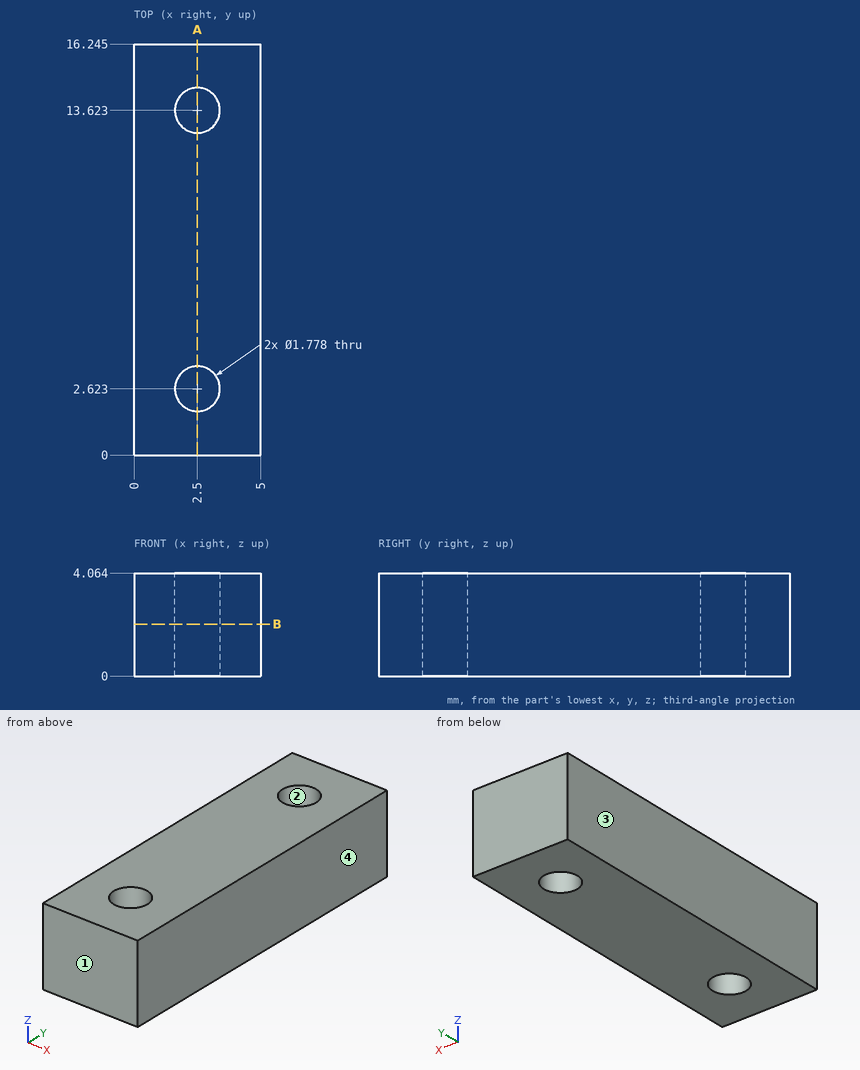
Source: three-view drawing plus pictorial views. Frame: mm from the lowest corner of the part. Give positions to 0.01 mm unless a question says otherwise; leave off trailing zeros. Write each loop counter-clockwise with the first axis right and the second up, starting at its lowest first coordinate (ties: lowest second). Pieces come first, ordered by that corner, then holes. Notation, with made-up numbers: (-23, -31) -> (4, -31) arc R13 cw to (4, -7) -> close; hole circle Ø3 at (17, -34.75). An arc over 180 degrees is marked (long way). Answer in a Markdown table with one row per item.
(1) Draft query along X for the marked faces 1, 2, 3 and 4. Return one class per face: +X half, -X half, draft (parallel to the pull), parting line (faces both ways), or undercut.
Answers below:
| item | result |
|---|---|
| face 1 | draft |
| face 2 | undercut |
| face 3 | -X half |
| face 4 | +X half |
(2) Section query A-A on x = 2.5. Return loops of the section in (y, z) (1 decimal).
Answers below:
| item | result |
|---|---|
| outline | (0, 0) -> (1.7, 0) -> (1.7, 4.1) -> (0, 4.1) -> close; (3.5, 0) -> (12.7, 0) -> (12.7, 4.1) -> (3.5, 4.1) -> close; (14.5, 0) -> (16.2, 0) -> (16.2, 4.1) -> (14.5, 4.1) -> close |
(3) Ray query, line 1 along Y through (x, z) = (2.5, 2.25) (1 decimal); line 2 along Y through (x, z) = (2.7, 1.65) (1 decimal); line 3 along X through (y, z) = (13.75, 3.55). Return the intervals inside material, ascending. Write a range as [from, to].
Answers below:
| item | result |
|---|---|
| line 1 | [0, 1.7], [3.5, 12.7], [14.5, 16.2] |
| line 2 | [0, 1.8], [3.5, 12.8], [14.5, 16.2] |
| line 3 | [0, 1.62], [3.38, 5] |
(4) Section query B-B on z = 2.05. Return loops of the section in (x, y) (1 decimal).
Answers below:
| item | result |
|---|---|
| outline | (0, 0) -> (5, 0) -> (5, 16.2) -> (0, 16.2) -> close; hole circle Ø1.8 at (2.5, 2.6); hole circle Ø1.8 at (2.5, 13.6) |
